Here's how the part is built. I have some questions about the finished solid (model axes, mm). A direction names the side the tool comes from. Round coordinates to 2 decimals unless told otherwise and drop trailing zeros. Loops run counter-clockwise (first coordinate to the right, second up) from the corner with the lowest first, then second, coordinate; pieces in that order, holes last. Notation, with made-up numbers: M 72.25,74.25 L 108.25,74.25 A5 ccw 108.25,81.25 Z; hole C 57.5,71 d7. An arc over 180 degrees is marked long. Use a Markdown table: item, result.
from build123d import *

# Parameters (mm, degrees)
BOX012_W               = 16
BOX012_H               = 4
BOX012_DEPTH           = 43
BOX012_PLACEMENT_ANGLE = 22
BOX011_W               = 16
BOX011_H               = 4
BOX011_DEPTH           = 43
BOX011_PLACEMENT_ANGLE = 22
BOX008_W               = 13
BOX008_H               = 4
BOX008_DEPTH           = 34
BOX009_W               = 13
BOX009_H               = 4
BOX009_DEPTH           = 34
BOX010_W               = 13
BOX010_H               = 4
BOX010_DEPTH           = 10
BOX007_W               = 39
BOX007_H               = 4
BOX007_DEPTH           = 14


with BuildPart() as obj1:
    # Box012 → Box012 (new body)
    with BuildSketch(Plane.XY):
        with Locations((8, 2)):
            Rectangle(BOX012_W, BOX012_H)
    extrude(amount=BOX012_DEPTH)


with BuildPart() as obj1_1:
    # Box012 placement: moved
    add(obj1.part.moved(Location((42, 0, 8))).rotate(Axis((42, 0, 8), (0, -1, 0)), BOX012_PLACEMENT_ANGLE))


with BuildPart() as fusion008:
    # Box011 → Box011 (new body)
    with BuildSketch(Plane.XY):
        with Locations((8, 2)):
            Rectangle(BOX011_W, BOX011_H)
    extrude(amount=BOX011_DEPTH)


with BuildPart() as fusion008_1:
    # Box011 placement: moved
    add(fusion008.part.moved(Location((-18, 0, 14))).rotate(Axis((-18, 0, 14), (0, 1, 0)), BOX011_PLACEMENT_ANGLE))

    # Fusion008: union obj1
    add(obj1_1.part)


with BuildPart() as obj2:
    # Box008 → Box008 (new body)
    with BuildSketch(Plane.XY.offset(14)):
        with Locations((6.5, 2)):
            Rectangle(BOX008_W, BOX008_H)
    extrude(amount=BOX008_DEPTH)


with BuildPart() as obj3:
    # Box009 → Box009 (new body)
    with BuildSketch(Plane(origin=(26, 0, 14), x_dir=(1, 0, 0), z_dir=(0, 0, 1))):
        with Locations((6.5, 2)):
            Rectangle(BOX009_W, BOX009_H)
    extrude(amount=BOX009_DEPTH)


with BuildPart() as obj4:
    # Box010 → Box010 (new body)
    with BuildSketch(Plane(origin=(13, 0, 38), x_dir=(1, 0, 0), z_dir=(0, 0, 1))):
        with Locations((6.5, 2)):
            Rectangle(BOX010_W, BOX010_H)
    extrude(amount=BOX010_DEPTH)


with BuildPart() as cut003:
    # Box007 → Box007 (new body)
    with BuildSketch(Plane.XY):
        with Locations((19.5, 2)):
            Rectangle(BOX007_W, BOX007_H)
    extrude(amount=BOX007_DEPTH)

    # Fusion007: union obj2, obj3, obj4
    add(obj2.part)
    add(obj3.part)
    add(obj4.part)

    # Cut003: cut Fusion008
    add(fusion008_1.part, mode=Mode.SUBTRACT)


with BuildPart() as cut003_1:
    # Cut003 placement: moved
    add(cut003.part.moved(Location((21, 8, -7))))


solid = cut003_1.part
1. Which directions (+Z, -Z, +X, -X, +Y, -Y) give clear straight access to the entire face, cutting with the end or side of a thin tool? Please do faces 4 (the face through (60, 10, 1)), 5 (the face through (40, 10, 7)).
Answer sheet:
| item | result |
|---|---|
| face 4 | +Z, -Z, +X, +Y, -Y |
| face 5 | +Y, -Y |
2. I need wall thicknesses on probe 1 along Z at (x, y) = (45, 11.75); probe 2 along X at (y, z) = (10.55, 12); probe 3 along X at (y, z) = (10.1, 29). Which ranges of each line are inside material? Lowest first, please. Write a range as from..to.
Answer sheet:
| item | result |
|---|---|
| probe 1 | -7..7, 31..41 |
| probe 2 | 22.28..34, 47..58.56 |
| probe 3 | 29.15..34, 47..51.69 |
3. Imagine slicing it at D-D, the plane x = 50. Write out the boundary of the cut face in (y, z).
Answer sheet:
| item | result |
|---|---|
| outline | M 8,-7 L 12,-7 L 12,33.18 L 8,33.18 Z |
4. Imagine slicing it at B-B, the plane x = 44. Write out the boundary of the cut face in (y, z).
Answer sheet:
| item | result |
|---|---|
| outline | M 8,-7 L 12,-7 L 12,7 L 8,7 Z; M 8,31 L 12,31 L 12,41 L 8,41 Z |
5. Imagine slicing it at C-C, the plane z = 16. Write out the boundary of the cut face in (x, y).
Answer sheet:
| item | result |
|---|---|
| outline | M 23.89,8 L 34,8 L 34,12 L 23.89,12 Z; M 47,8 L 56.94,8 L 56.94,12 L 47,12 Z |
6. We'd pull the mould along Z, two halves only. Please class faces 1 (the face through (34, 10, 19)), 2 (the face through (40, 8, 6)), 3 (the face through (40, 10, 41)): +Z half, -Z half, draft (parallel to the pull), parting line (faces both ways), or undercut.
Answer sheet:
| item | result |
|---|---|
| face 1 | undercut |
| face 2 | draft |
| face 3 | +Z half |
7. Imagine slicing it at A-A, the plane y = 11.1. Write out the boundary of the cut face in (x, z), then the cut area to 3 significant figures.
Answer sheet:
| item | result |
|---|---|
| outline | M 21,-7 L 60,-7 L 60,8.43 L 46.89,40.87 L 47.22,41 L 33.63,41 L 33.94,40.88 L 21,8.84 Z; hole M 34,7 L 47,7 L 47,31 L 34,31 Z |
| area | 1,140 mm2 |
8. For pin 1 Ø1.5 at (y, z) = (9, 26) entering from -X, with a flat end and sliding along its axis, tell me the tip position at first contact or that it passes through.
Answer sheet:
| item | result |
|---|---|
| pin 1 | x = 27.63 |
